Autodesk Inventor part; units mm, degrees
ref_plane "YZ Plane" through (0, 0, 0) normal (1, 0, 0) x (0, 1, 0)
ref_plane "XZ Plane" through (0, 0, 0) normal (0, 1, 0) x (-1, 0, 0)
ref_plane "XY Plane" through (0, 0, 0) normal (0, 0, 1) x (1, 0, 0)
sketch "Sketch1" plane through (0, 0, 0) normal (0, 0, 1) x (1, 0, 0)
  arc A0 (-94.4262, -10.1366) -> (-94.4262, 9.3452) centre (-94.4262, -0.3957) ccw
  arc A1 (-260.35, 9.3452) -> (-260.35, -10.1366) centre (-260.35, -0.3957) ccw
  line L0 (-260.35, 9.3452) -> (-94.4262, 9.3452)
  line L1 (-94.4262, -10.1366) -> (-260.35, -10.1366)
  circle A2 centre (-260.35, -0.3957) radius 3.2512
  circle A3 centre (-94.4262, -0.3957) radius 3.2512
  circle A4 centre (-171.45, -0.3957) radius 3.2512
  line L2 (-260.35, -0.3957) -> (-260.35, 9.3452) construction
  dimension "d0" = 19.4818
  dimension "d1" = 19.4818
  dimension "d3" = 6.5024
  dimension "d4" = 6.5024
  dimension "d12" = 6.5024
  dimension "d13" = 9.7409
  dimension "d14" = 88.9
  dimension "d19" = 90
extrude "Extrusion1" add sketch "Sketch1" along normal blind 2.54
equation "\"d0\" = d1"
properties part number "ArmConnector1"
Can you work these out from the model? Positions are in its coordinate system, mm. Coordinates: 2 decimals unless noted, no trailing zeros. Write each loop counter-clockwise with the first axis right and the second up, starting at its lowest first coordinate (ties: lowest second). Pieces come first, ordered by that corner, then holes. Notation, with made-up numbers: (-26.5, 42) -> (3.5, 42) arc R26 cw to (3.5, 71) -> close; hole circle Ø5 at (-26, 16.5). An arc over 180 degrees is marked (long way). Write each question's results on one line, items separated by ' | '. Start each with the question number.
Q1. I'm going to push a flat-ended pin straight in: pin 1 (1.5 mm diameter, centred on y = 5.5, z = 2, fed in from +X). Where does the tip first touch, or does it pass through?
Q2. Imagine slicing it at C-C (y = 7). Write out the boundary of the cut face in (x, z).
Q3. Imagine slicing it at B-B (z = 1.6). Write out the boundary of the cut face in (x, y) (3 decimals).
Q4. Imagine slicing it at A-A (x = -171.45). Write out the boundary of the cut face in (y, z), then the cut area to 3 significant figures.
Q5. We'd pull the mould along X, two halves only. Please class faces 1 (the face through (-84.688, -0.182, 1.252)), 2 (the face through (-263.6, -0.5, 1.3)), 3 (the face through (-179, 0, 0)): +X half, -X half, draft (parallel to the pull), parting line (faces both ways), or undercut.
Q6. If I drill on probe 1 along X at (y, z) = (-0.5, 0.2); probe 2 along Y at (x, z) = (-171.45, 1.3); probe 3 along X at (y, z) = (-6, 1.7), over which ranges is the centre line in solid material (lowest first)?
Taken from the geometry:
1) pin 1: stops at x = -86.16
2) outline: (-266.69, 0) -> (-88.09, 0) -> (-88.09, 2.54) -> (-266.69, 2.54) -> close
3) outline: (-260.35, -10.137) -> (-94.426, -10.137) arc R9.741 ccw to (-94.426, 9.345) -> (-260.35, 9.345) arc R9.741 ccw to start; hole circle Ø6.502 at (-260.35, -0.396); hole circle Ø6.502 at (-171.45, -0.396); hole circle Ø6.502 at (-94.426, -0.396)
4) outline: (-10.14, 0) -> (-3.65, 0) -> (-3.65, 2.54) -> (-10.14, 2.54) -> close; (2.86, 0) -> (9.35, 0) -> (9.35, 2.54) -> (2.86, 2.54) -> close | area: 33.0 mm^2
5) face 1: +X half | face 2: undercut | face 3: draft
6) probe 1: x = -270.09 to -263.6, -257.1 to -174.7, -168.2 to -97.68, -91.18 to -84.69 | probe 2: y = -10.14 to -3.65, 2.86 to 9.35 | probe 3: x = -268.32 to -86.46
